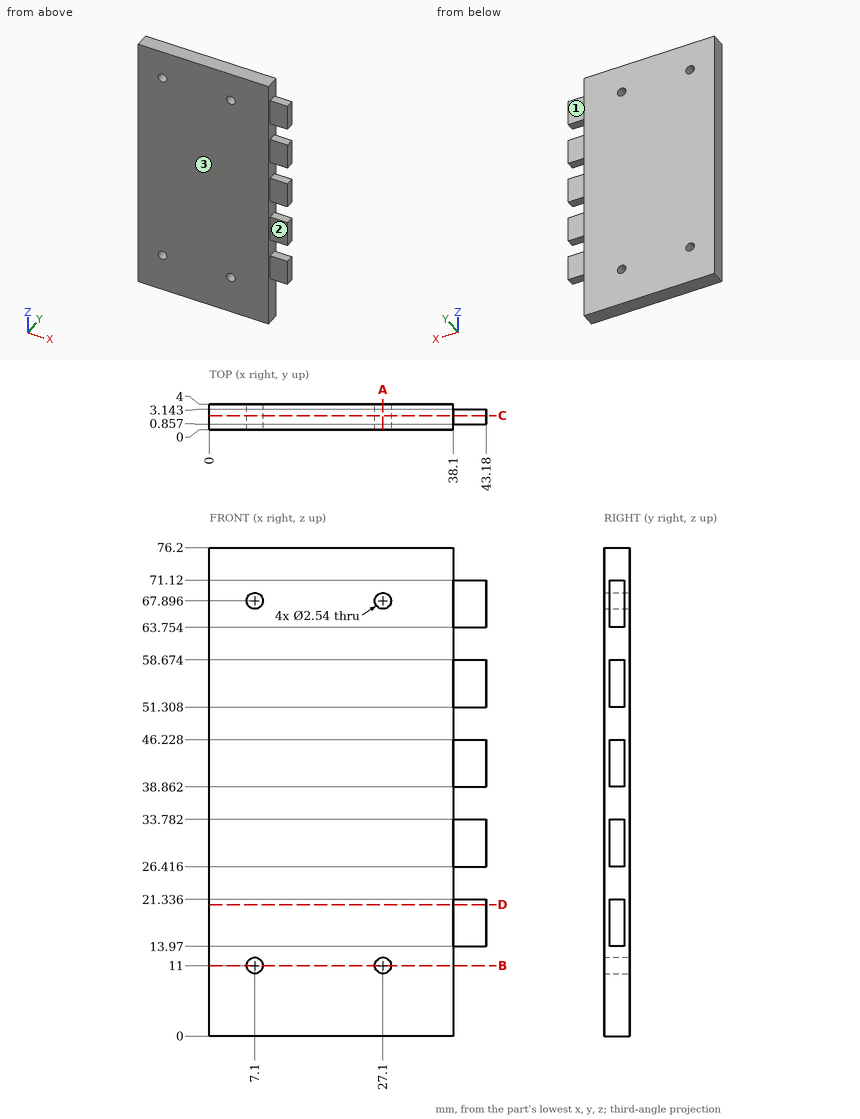
Verification items for this drawing (mm, ordinates from the low corner). A direction names the side the tool comes from. Coordinates: 2 decimals unless noted, no trailing zeros. Write each loop counter-clockwise with the first axis right and the second up, starting at its lowest first coordinate (ties: lowest second). Pieces come first, ordered by that corner, then holes. Notation, with made-up numbers: M 9,68.25 L 66,68.25 A14 ccw 66,80.25 Z; hole C -11.5,-30 d5. An arc over 180 degrees is marked long. Use one line per item in the form item = value. Start each with the question number.
1) Section check C-C on y = 2.2. Enter the section's corners in (x, z), and give its area (3 significant figures).
2) Go/stop test with flat-tipped pins: pin 1 Ø1.5 at (x, z) = (41, 65.5) entering from +Y; pin 2 Ø0.7 at (x, y) = (42, 2.5) entering from -Z; pin 3 Ø0.7 at (x, y) = (40.5, 2.5) entering from +Z. Record where each tip stops, or that it passes through.
3) Thickness scan on probe 1 along X at (y, z) = (1.8, 11); probe 2 along Z at (x, y) = (7.1, 3); probe 3 along X at (y, z) = (1.4, 37.5). Record the ranges inside material, lowest first. Write a range as from..to.
4) Section check D-D on z = 20.5. Enter the section's corners in (x, y).
5) Section check A-A on x = 27.1. Enter the section's corners in (y, z), and give its area (3 significant figures).
6) Set-up check for the marked faces 1, 2 and 3: record each of +Z, -Z, +X, -X, +Y, -Y from which the full face is reachable in a straight line by a thin tool's end or side.
7) Section check B-B on z = 11. Enter the section's corners in (x, y), and give its area (3 significant figures).
Responses:
q1.outline = M 0,0 L 38.1,0 L 38.1,13.97 L 43.18,13.97 L 43.18,21.34 L 38.1,21.34 L 38.1,26.42 L 43.18,26.42 L 43.18,33.78 L 38.1,33.78 L 38.1,38.86 L 43.18,38.86 L 43.18,46.23 L 38.1,46.23 L 38.1,51.31 L 43.18,51.31 L 43.18,58.67 L 38.1,58.67 L 38.1,63.75 L 43.18,63.75 L 43.18,71.12 L 38.1,71.12 L 38.1,76.2 L 0,76.2 Z; hole C 7.1,11 d2.54; hole C 7.1,67.9 d2.54; hole C 27.1,11 d2.54; hole C 27.1,67.9 d2.54
q1.area = 3,070 mm2
q2.pin_1 = 3.14
q2.pin_2 = 13.97
q2.pin_3 = 71.12
q3.probe_1 = 0..5.83, 8.37..25.83, 28.37..38.1
q3.probe_2 = 0..9.73, 12.27..66.63, 69.17..76.2
q3.probe_3 = 0..38.1
q4.outline = M 0,0 L 38.1,0 L 38.1,0.86 L 43.18,0.86 L 43.18,3.14 L 38.1,3.14 L 38.1,4 L 0,4 Z
q5.outline = M 0,0 L 4,0 L 4,9.73 L 0,9.73 Z; M 0,12.27 L 4,12.27 L 4,66.63 L 0,66.63 Z; M 0,69.17 L 4,69.17 L 4,76.2 L 0,76.2 Z
q5.area = 284 mm2
q6.face_1 = +Z, -Z, +X, +Y
q6.face_2 = +Z, -Z, +X, -Y
q6.face_3 = +Z, -Z, +X, -X, -Y
q7.outline = M 0,0 L 5.83,0 L 5.83,4 L 0,4 Z; M 8.37,0 L 25.83,0 L 25.83,4 L 8.37,4 Z; M 28.37,0 L 38.1,0 L 38.1,4 L 28.37,4 Z
q7.area = 132 mm2
